```python
from build123d import *

# Parameters (mm, degrees)
BOSS_EXTRUDE1_DEPTH = 9
CUT_EXTRUDE1_DEPTH  = 3
SKETCH5_W           = 6
SKETCH5_H           = 5
CUT_EXTRUDE2_DEPTH  = 6


with BuildPart() as part:
    # Sketch1 → Boss-Extrude1 (new body)
    with BuildSketch(Plane(origin=(0, 0, 0), x_dir=(0, 0, -1), z_dir=(1, 0, 0))):
        with BuildLine():
            Line((-4.5, -5), (4.5, -5))
            Line((4.5, -5), (4.5, -3))
            Line((4.5, -3), (3.5, -3))
            Line((3.5, -3), (3.5, 3))
            Line((3.5, 3), (4.5, 3))
            Line((4.5, 3), (4.5, 5))
            Line((4.5, 5), (-4.5, 5))
            Line((-4.5, 5), (-4.5, 3))
            ThreePointArc((-4.5, 3), (-2.378679656, 2.121320344), (-1.5, 0))
            ThreePointArc((-1.5, 0), (-2.378679656, -2.121320344), (-4.5, -3))
            Line((-4.5, -3), (-4.5, -5))
        make_face()
    extrude(amount=BOSS_EXTRUDE1_DEPTH)

    # Sketch3 → Cut-Extrude1 (cut)
    with BuildSketch(Plane(origin=(9, 0, 0), x_dir=(0, 0, -1), z_dir=(1, 0, 0))):
        with BuildLine():
            ThreePointArc((-4.5, 3), (-2.378679656, 2.121320344), (-1.5, 0))
            Line((-1.5, 0), (0.5, 0))
            Line((0.5, 0), (0.5, 5))
            Line((0.5, 5), (-4.5, 5))
            Line((-4.5, 5), (-4.5, 3))
        make_face()
        Polygon((1.5, -1), (1.5, -5), (4.5, -5), (4.5, -3), (3.5, -3), (3.5, -1), align=None)
    extrude(amount=-CUT_EXTRUDE1_DEPTH, mode=Mode.SUBTRACT)

    # Sketch5 → Cut-Extrude2 (cut)
    with BuildSketch(Plane(origin=(9, 0, 0), x_dir=(0, 0, -1), z_dir=(1, 0, 0))):
        with Locations((-1.5, -2.5)):
            Rectangle(SKETCH5_W, SKETCH5_H)
    extrude(amount=-CUT_EXTRUDE2_DEPTH, mode=Mode.SUBTRACT)


solid = part.part
```
Model file for the job. Use its own axes, mm. A direction names the side the tool comes from. Coordinates: 2 decimals unless noted, no trailing zeros. Order: outer loops, then holes, each group sorted by start corner. A loop starts at its lowest first (then second) coordinate and runs counter-clockwise, first axis right, second up. Notation, with made-up numbers: (37, -11) -> (95, -11) arc R23 ccw to (95, 25) -> close; hole circle Ø11 at (16.25, 86.5). An arc over 180 degrees is marked (long way). Return JSON: item names as keys, results as strings.
Item 1: Pin check, flat tips, straight feed: P1, Ø4, axis at y = 1.5, z = 2.5, coming from the +X side; P2, Ø1.5, axis at y = -2.5, z = 0.5, coming from the +X side; P3, Ø2.5, axis at x = 5, z = 0, coming from the -Y side. Stop position of each tip, or through.
Model answer:
{"P1": "stops at x = 6", "P2": "stops at x = 3", "P3": "stops at y = 0"}
Item 2: Mould opens along Y. For faces 5 (the face through (4, 0, -3.5)), 6 (the face through (3, 5, 0)), 7 (the face through (8, -1, -3)), 8 (the face through (4, 4, -4.5)) say: pulls with the +Y half, pulls with the -Y half, needs draft (parallel to the pull), parting line crosses it, or undercut.
Model answer:
{"face 5": "undercut", "face 6": "pulls with the +Y half", "face 7": "pulls with the -Y half", "face 8": "needs draft"}
Item 3: Slice it at C-C (y = -4.5). Write the cut outline in (x, z).
Model answer:
{"outline": "(0, -4.5) -> (6, -4.5) -> (6, -1.5) -> (3, -1.5) -> (3, 4.5) -> (0, 4.5) -> close"}
Item 4: Slice it at A-A (x = 1.75). Write the cut outline in (y, z).
Model answer:
{"outline": "(-5, -4.5) -> (-3, -4.5) -> (-3, -3.5) -> (3, -3.5) -> (3, -4.5) -> (5, -4.5) -> (5, 4.5) -> (3, 4.5) arc R3 cw to (-3, 4.5) -> (-5, 4.5) -> close"}
Item 5: Slice it at D-D (z = 0). Write the cut outline in (x, y), then the cut area to 3 significant figures.
Model answer:
{"outline": "(0, -5) -> (3, -5) -> (3, 0) -> (6, 0) -> (6, 5) -> (0, 5) -> close", "area": "45.0 mm²"}
Item 6: Slice it at B-B (z = 3.75). Write the cut outline in (x, y).
Model answer:
{"outline": "(0, -5) -> (3, -5) -> (3, -2.9) -> (0, -2.9) -> close; (0, 2.9) -> (6, 2.9) -> (6, 5) -> (0, 5) -> close"}
Item 7: 3-axis set-ups, long thin cutter, end or side, ignore diameter. For faces 1 (the face through (6, -3, -3)), 2 (the face through (4, 3, -4)), 3 (the face through (5, -2, -1.5)), 4 (the face through (8, 2, -0.5)): which of +Z, -Z, +X, -X, +Y, -Y reach the whole face in a straight line?
Model answer:
{"face 1": "+Z, -Z, +X, -Y", "face 2": "-Z, +X, -X", "face 3": "+Z, +X, -Y", "face 4": "+Z, +X, +Y, -Y"}
Item 8: Wall check: line 1 along X through (y, z) = (-3, 2.75); line 2 along X through (y, z) = (1.75, 1.25); line 3 along Y through (x, z) = (1, 2.5). Give the ranges that are in metal, low to high. Write a range as from..to.
Model answer:
{"line 1": "x = 0..3", "line 2": "x = 0..6", "line 3": "y = -5..-2.24, 2.24..5"}
